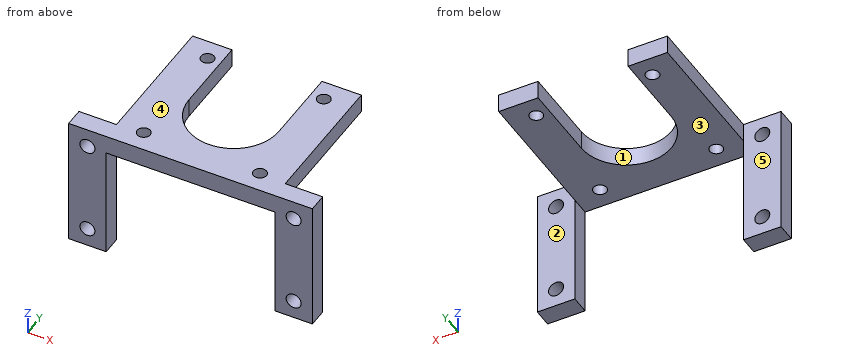
from build123d import *

# Parameters (mm, degrees)
ESBO_O1_R                = 1.75
RESSALTO_EXTRUS_O1_DEPTH = 5
ESBO_O2_W                = 10
ESBO_O2_H                = 35
ESBO_O2_R                = 2
RESSALTO_EXTRUS_O2_DEPTH = 5


with BuildPart() as part:
    # Esboço1 → Ressalto-extrusão1 (new body)
    with BuildSketch(Plane.XY):
        with BuildLine():
            Line((-12, 0), (-12, 21))
            Line((-12, 21), (-22.5, 21))
            Line((-22.5, 21), (-22.5, -21))
            Line((-22.5, -21), (22.5, -21))
            Line((22.5, -21), (22.5, 21))
            Line((22.5, 21), (12, 21))
            Line((12, 21), (12, 0))
            ThreePointArc((12, 0), (0, -12), (-12, 0))
        make_face()
        with Locations((-15.5, 15.5)):
            Circle(ESBO_O1_R, mode=Mode.SUBTRACT)
        with Locations((15.5, 15.5)):
            Circle(ESBO_O1_R, mode=Mode.SUBTRACT)
        with Locations((15.5, -15.5)):
            Circle(ESBO_O1_R, mode=Mode.SUBTRACT)
        with Locations((-15.5, -15.5)):
            Circle(ESBO_O1_R, mode=Mode.SUBTRACT)
    extrude(amount=RESSALTO_EXTRUS_O1_DEPTH)

    # Esboço2 → Ressalto-extrusão2 (add)
    # profile 1 of 2: a face of its own
    with BuildSketch(Plane.XZ.offset(21)):
        with Locations((-27.5, -12.5)):
            Rectangle(ESBO_O2_W, ESBO_O2_H)
        with Locations(Location((-27.5, -25, 0), (0, 0, 270))):
            Circle(ESBO_O2_R, mode=Mode.SUBTRACT)
        with Locations(Location((-27.5, 0, 0), (0, 0, 270))):
            Circle(ESBO_O2_R, mode=Mode.SUBTRACT)
    # profile 2 of 2: a face of its own
    with BuildSketch(Plane.XZ.offset(21)):
        with Locations((27.5, -12.5)):
            Rectangle(ESBO_O2_W, ESBO_O2_H)
        with Locations(Location((27.5, 0, 0), (0, 0, 90))):
            Circle(ESBO_O2_R, mode=Mode.SUBTRACT)
        with Locations(Location((27.5, -25, 0), (0, 0, 90))):
            Circle(ESBO_O2_R, mode=Mode.SUBTRACT)
    extrude(amount=-RESSALTO_EXTRUS_O2_DEPTH)


solid = part.part
Work out the finished part from the listing and answer in its coordinate system (mm). Face numbers are marked on the shaded views. A direction names the side the tool comes from. Round coordinates to 2 decimals unless told otherwise and drop trailing zeros. Write each loop counter-clockwise with the first axis right and the second up, starting at its lowest first coordinate (ties: lowest second). Pieces come first, ordered by that corner, then holes.
1) Straight lines are drawn through the part: line 1 (Y direction, x = 15.5, z = 2.45); line 2 (X direction, y = 15, z = 3); line 3 (X direction, y = -15, z = 1). For each, find the intervals that lie inside material, in ascending order.
2) A tool of negligible diameter and unlimited length cuts with its end or side. For the marked faces 3, 4 and 5, from which of +Z, -Z, +X, -X, +Y, -Y can it reach the whole face along a straight path? Write none if from no direction.
3) A cutting plane is placed at B-B (z = -25). Give the vertices of the cut face in (x, y).
4) A cutting plane is placed at A-A (x = 15.5). Give the vertices of the cut face in (y, z).
5) The mould has two halves that part along X. Classify the marked faces 1 and 2: pulls with the +X half, pulls with the -X half, needs draft (parallel to the pull), parting line crosses it, or undercut.
6) Given pin 1 Ø12 at (y, z) = (-2.5, -1) entering from +X; pin 2 Ø10 at (x, y) = (-17.5, 14) entering from -Z; pin 3 Ø6.5 at (x, z) = (-27.5, -25) entering from +Y; pin 4 Ø8 at (x, y) = (25.5, -14.5) entering from +Z, each flat-ended and moving along its own axis, determine where each tip first touches the part or whether it passes through.
7) A cutting plane is placed at C-C (y = 1.5). Give the vertices of the cut face in (x, z).
8) A cutting plane is placed at D-D (z = -18.5). Give the vertices of the cut face in (x, y), plus the area to 3 significant figures.
Completed:
1. line 1: y = -21 to -17.25, -13.75 to 13.75, 17.25 to 21
1. line 2: x = -22.5 to -17.18, -13.82 to -12, 12 to 13.82, 17.18 to 22.5
1. line 3: x = -22.5 to -17.18, -13.82 to 13.82, 17.18 to 22.5
2. face 3: -Z, +Y, -Y
2. face 4: +Z, +X, -X, +Y, -Y
2. face 5: +Z, -Z, -X, +Y
3. outline: (-32.5, -21) - (-29.5, -21) - (-29.5, -16) - (-32.5, -16) - close; (-25.5, -21) - (-22.5, -21) - (-22.5, -16) - (-25.5, -16) - close; (22.5, -21) - (25.5, -21) - (25.5, -16) - (22.5, -16) - close; (29.5, -21) - (32.5, -21) - (32.5, -16) - (29.5, -16) - close
4. outline: (-21, 0) - (-17.25, 0) - (-17.25, 5) - (-21, 5) - close; (-13.75, 0) - (13.75, 0) - (13.75, 5) - (-13.75, 5) - close; (17.25, 0) - (21, 0) - (21, 5) - (17.25, 5) - close
5. face 1: undercut
5. face 2: needs draft
6. pin 1: stops at x = 22.5
6. pin 2: stops at z = 0
6. pin 3: stops at y = -16
6. pin 4: stops at z = 5
7. outline: (-22.5, 0) - (-12, 0) - (-12, 5) - (-22.5, 5) - close; (12, 0) - (22.5, 0) - (22.5, 5) - (12, 5) - close
8. outline: (-32.5, -21) - (-22.5, -21) - (-22.5, -16) - (-32.5, -16) - close; (22.5, -21) - (32.5, -21) - (32.5, -16) - (22.5, -16) - close
8. area: 100 mm2
